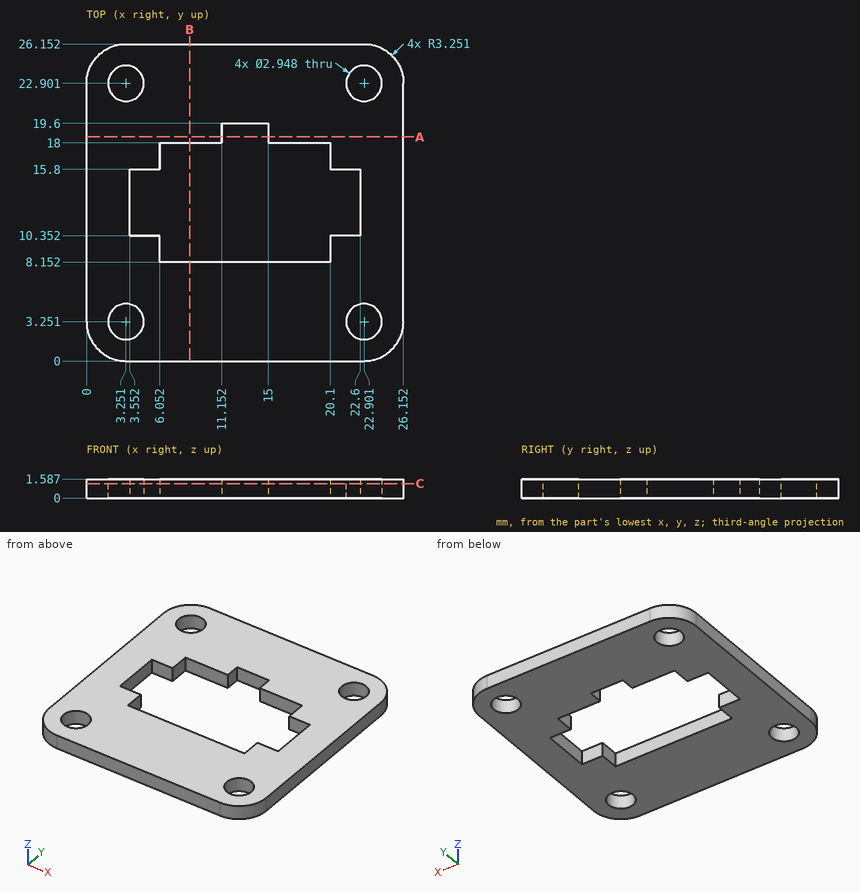
Input: dimensioned drawing with shaded views. Units: mm. Origin: part minimum x, y, z. Give positions to 0.01 mm unless a question says otherwise; leave off trailing zeros. Write each loop counter-clockwise with the first axis right and the second up, starting at its lowest first coordinate (ties: lowest second). Pieces come first, ordered by that corner, then holes. Notation, with made-up numbers: M 54,35 L 92,35 A27 ccw 92,55 Z; hole C 11.5,85.5 d1. An arc over 180 degrees is marked long. Return JSON: item names as keys, results as strings. Group by question number.
1) Cut plane C-C, the plane z = 1.2. Output: boundary loops of the cut face in (x, y) (1 decimal), plus the area to 3 significant figures.
2) Pin query (flat end, axial travel): P1, Ø6, axis at x = 14.5, y = 13, coming from the -Z side (3 decimals). Return the tip coordinate at first contact, or that it passes through.
3) Material intervals for line 1 along X through (y, z) = (9.5, 1.25); line 2 along X through (y, z) = (18.5, 1.25); line 3 along Y through (x, z) = (20.75, 1), sorted ascending. Write a range as [from, to].
4) Cut plane A-A, the plane y = 18.5. Output: boundary loops of the cut face in (x, z).
5) Cut plane B-B, the plane x = 8.5. Output: boundary loops of the cut face in (y, z).
Recorded:
{
 "1": {"outline": "M 0,3.3 A3.3 ccw 3.3,0 L 22.9,0 A3.3 ccw 26.2,3.3 L 26.2,22.9 A3.3 ccw 22.9,26.2 L 3.3,26.2 A3.3 ccw 0,22.9 Z; hole C 3.3,3.3 d2.9; hole C 3.3,22.9 d2.9; hole M 3.6,10.4 L 6.1,10.4 L 6.1,8.2 L 20.1,8.2 L 20.1,10.4 L 22.6,10.4 L 22.6,15.8 L 20.1,15.8 L 20.1,18 L 15,18 L 15,19.6 L 11.2,19.6 L 11.2,18 L 6.1,18 L 6.1,15.8 L 3.6,15.8 Z; hole C 22.9,3.3 d2.9; hole C 22.9,22.9 d2.9", "area": "476 mm²"},
 "2": {"P1": "passes through"},
 "3": {"line 1": "x = [0, 6.05], [20.1, 26.15]", "line 2": "x = [0, 11.15], [15, 26.15]", "line 3": "y = [0, 10.35], [15.8, 26.15]"},
 "4": {"outline": "M 0,0 L 11.15,0 L 11.15,1.59 L 0,1.59 Z; M 15,0 L 26.15,0 L 26.15,1.59 L 15,1.59 Z"},
 "5": {"outline": "M 0,0 L 8.15,0 L 8.15,1.59 L 0,1.59 Z; M 18,0 L 26.15,0 L 26.15,1.59 L 18,1.59 Z"}
}
